from build123d import *

# Parameters (mm, degrees)
PAD_DEPTH       = 3
SKETCH001_W     = 2
SKETCH001_H     = 6
POCKET_DEPTH    = 5
PAD001_DEPTH    = 2.2
SKETCH003_R     = 1.571244
POCKET001_DEPTH = 5


with BuildPart() as part:
    # Sketch → Pad (new body)
    with BuildSketch(Plane.XY):
        Polygon((0, -50), (9.32, -50), (9.32, 40), (35, 55), (35, 120), (0, 120), align=None)
    extrude(amount=PAD_DEPTH)

    # Sketch001 (on Face7 of Pad) → Pocket (cut)
    with BuildSketch(Plane(origin=(0, 0, 0), x_dir=(1, 0, 0), z_dir=(0, 0, -1))):
        with Locations((1, 0)):
            Rectangle(SKETCH001_W, SKETCH001_H)
    extrude(amount=-POCKET_DEPTH, mode=Mode.SUBTRACT)

    # Sketch002 (on Face3 of Pocket) → Pad001 (join)
    with BuildSketch(Plane.YZ.offset(9.32)):
        Polygon((-3, 0), (-3, 40), (-12, 40), (-34, 0), align=None)
    extrude(amount=PAD001_DEPTH)

    # Sketch003 (on Face18 of Pad001) → Pocket001 (cut)
    with BuildSketch(Plane.YZ.offset(11.52)):
        with Locations((-8.751605, 34.485332)):
            Circle(SKETCH003_R)
    extrude(amount=-POCKET001_DEPTH, mode=Mode.SUBTRACT)


solid = part.part
The listing builds one solid part. Answer for the finished solid, in the listing's coordinates (mm). A direction names the side the tool comes from. Coordinates: 2 decimals unless noted, no trailing zeros. Loops run counter-clockwise (first coordinate to the right, second up) from the corner with the lowest first, then second, coordinate; pieces in that order, holes last.
1) Find section C-C on y = -29. Write down the section's boundary in (x, z).
2) Find the intervals of material crossed by L1, parallel to Z at x = 13.5, y = 98.5; L2, parallel to X at y = -10.5, z = 4.5; L3, parallel to Y at x = 9.5, z = 20, in increasing order.
3) Find section A-A on z = 23. Write down the section's boundary in (x, y), then the cut area to 3 significant figures.
4) Find section B-B on y = 17. Write down the section's boundary in (x, z), then the cut area to 3 significant figures.
5) A tool of negligible diameter and unlimited length cuts with its end or side. For faces 1 (the face through (9.32, 18, 1)), 2 (the face through (9.32, -15, 18)), 3 (the face through (11.52, -15, 16)), 4 (the face through (2, 0, 1)), from which of +Z, -Z, +X, -X, +Y, -Y can it reach the whole face along a straight path? Write none if from no direction.
6) Flat-ended cylindrical pins translate along their axes: pin 1 Ø3 at (x, z) = (13.5, 32.5) entering from -Y; pin 2 Ø2.5 at (y, z) = (-1, 2) entering from -X; pin 3 Ø4 at (y, z) = (59, 4.5) entering from -X; pin 4 Ø9 at (y, z) = (-21.5, 13) entering from -X. Find the tip coordinate at first contact, or state that the pin passes through.
Values:
1. outline: (0, 0) - (11.52, 0) - (11.52, 9.09) - (9.32, 9.09) - (9.32, 3) - (0, 3) - close
2. L1: z = 0 to 3
2. L2: x = 9.32 to 11.52
2. L3: y = -23 to -3
3. outline: (9.32, -21.35) - (11.52, -21.35) - (11.52, -3) - (9.32, -3) - close
3. area: 40.4 mm2
4. outline: (0, 0) - (9.32, 0) - (9.32, 3) - (0, 3) - close
4. area: 28.0 mm2
5. face 1: +Z, -Z, +X
5. face 2: +Z, -X, +Y, -Y
5. face 3: +Z, -Z, +X, -Y
5. face 4: +Z, -Z, -X
6. pin 1: passes through
6. pin 2: stops at x = 2
6. pin 3: stops at x = 0
6. pin 4: stops at x = 9.32
